```python
from build123d import *

# Parameters (mm, degrees)
CUT_EXTRUDE1_DEPTH = 1.75


with BuildPart() as part:
    # Sketch2 → Revolve1 (revolve)
    with BuildSketch(Plane(origin=(0, 0, 0), x_dir=(0, 0, -1), z_dir=(1, 0, 0)), mode=Mode.PRIVATE) as revolve1_sk:
        with BuildLine():
            Line((-6.1, 0), (6.1, 0))
            Line((6.1, 0), (6.1, 1.44))
            Line((6.1, 1.44), (5.54, 2))
            Line((5.54, 2), (-3.9, 2))
            Line((-3.9, 2), (-3.9, 3.8))
            Line((-3.9, 3.8), (-4.23, 3.8))
            ThreePointArc((-4.23, 3.8), (-5.306499853, 3.047002626), (-6.1, 2))
            Line((-6.1, 2), (-6.1, 0))
        make_face()
    revolve(revolve1_sk.sketch.rotate(Axis((0, 0, 6.1), (0, 0, -1)), 90), axis=Axis((0, 0, 6.1), (0, 0, -1)))

    # Sketch3 → Cut-Extrude1 (cut)
    with BuildSketch(Plane.XY.offset(6.1)):
        Polygon((0, 1.443375673), (-1.25, 0.721687836), (-1.25, -0.721687836), (0, -1.443375673), (1.25, -0.721687836), (1.25, 0.721687836), align=None)
    extrude(amount=-CUT_EXTRUDE1_DEPTH, mode=Mode.SUBTRACT)

    # Cut-Extrude2 cone 1 section (through the dimple's axis) → Cut-Extrude2 (revolve, cut)
    with BuildSketch(Plane(origin=(0, 0, 6.1), x_dir=(0, -1, 0), z_dir=(1, 0, 0))):
        Polygon((0, 0), (1.443375673, 0), (0, 1.443375673), align=None)
    revolve(axis=Axis((0, 0, 6.1), (0, 0, -1)), mode=Mode.SUBTRACT)


solid = part.part
```
Geometry check sheet. Reference: the model listing, model coordinates, mm. A direction names the side the tool comes from. Round coordinates to 2 decimals unless told otherwise and drop trailing zeros. Order: outer loops, then holes, each group sorted by start corner. A loop starts at its lowest first (then second) coordinate and runs counter-clockwise, first axis right, second up. Notation, with made-up numbers: (5.5, 9) - (23.5, 9) arc R25 ccw to (23.5, 24) - close; hole circle Ø7 at (-19, -15.5). An arc over 180 degrees is marked (long way). Use a Markdown table: item, result. Add a question column.
1) Gauge pin test, flat ends, axial feed: P1, Ø4, axis at x = 3, z = -1.5, coming from the -Y side; P2, Ø0.7, axis at y = 0, z = 5.5, coming from the +X side; P3, Ø1, axis at y = 0, z = 0, coming from the -X side. Record the tip position at first contact, or that the pin passes through.
2) Section check C-C (x = -2.25). Record the cut outline in (y, z).
3) Mould release check, pull along Y, two halves, no side actions. Record for faces 1 (the cylindrical face through (3.625, -1.141, 4.067)), 2 (the flat face through (0, 0, 4.35)), 3 (the flat face through (-2, 2, 3.9)): released by +Y, released by -Y, zero draft, split by the parting line, or undercut.
4) Set-up check for faces 4 (the flat face through (0, 0, -6.1)), 5 (the flat face through (-0.616, 1.088, 5.237)), 6 (the cylindrical face through (0, 2, -1)): record each of +Z, -Z, +X, -X, +Y, -Y from which the full face is reachable in a straight line by a thin tool's end or side.
5) Section check D-D (y = -2.5). Record the cut outline in (x, z), then the cut area to 3 significant figures.
6) Section check A-A (z = 4.75). Record the cut outline in (x, y).
7) Section check B-B (z = 1.75). Record the cut outline in (x, y).
8) Thickness scan on line 1 along Z through (x, y) = (0.5, -1); line 2 along Y through (x, z) = (-0.25, 5); line 3 along Y through (x, z) = (-0.75, 2.5). Record the ranges inside material, lowest first.
Established:
| question | item | result |
|---|---|---|
| 1 | P1 | y = -1.73 |
| 1 | P2 | x = 3.19 |
| 1 | P3 | x = -2 |
| 2 | outline | (-3.06, 3.9) - (3.06, 3.9) - (3.06, 4.23) arc R3.58 ccw to (-3.06, 4.23) - close |
| 3 | face 1 | split by the parting line |
| 3 | face 2 | undercut |
| 3 | face 3 | zero draft |
| 4 | face 4 | -Z, +X, -X, +Y, -Y |
| 4 | face 5 | +Z |
| 4 | face 6 | -Z |
| 5 | outline | (-2.86, 3.9) - (2.86, 3.9) - (2.86, 4.23) arc R3.41 ccw to (-2.86, 4.23) - close |
| 5 | area | 8.16 mm2 |
| 6 | outline | circle Ø7 at (0, 0); hole (-1.25, -0.72) - (0, -1.44) - (1.25, -0.72) - (1.25, 0.72) - (0, 1.44) - (-1.25, 0.72) - close |
| 7 | outline | circle Ø4 at (0, 0) |
| 8 | line 1 | -6.1 to 4.35 |
| 8 | line 2 | -3.31 to -1.3, 1.3 to 3.31 |
| 8 | line 3 | -1.85 to 1.85 |
